The model under review builds one solid part; all positions refer to its coordinate system, in mm. Face numbers are marked on the shaded views. A direction names the side the tool comes from. Round coordinates to 2 decimals unless told otherwise and drop trailing zeros. Order: outer loops, then holes, each group sorted by start corner. A loop starts at its lowest first (then second) coordinate and runs counter-clockwise, first axis right, second up.
```python
from build123d import *

# Parameters (mm, degrees)
SKETCH1_R                   = 2.5
SKETCH1_R_2                 = 1
BOSS_EXTRUDE1_DEPTH         = 5
CHAMFER2_SIZE               = 4
CHAMFER2_SIZE2              = 0.705307923
LPATTERN2_COUNT             = 2
LPATTERN2_PITCH             = 5
CHAMFER2_OF_LPATTERN2_SIZE2 = 0.705307923
CHAMFER2_OF_LPATTERN2_SIZE  = 4
FILLET1_R                   = 1
SKETCH2_R                   = 10
BOSS_EXTRUDE2_DEPTH         = 15
CUT_EXTRUDE1_START          = -2
SKETCH3_R                   = 8
CUT_EXTRUDE1_DEPTH          = 15
CUT_EXTRUDE2_START          = -15
SKETCH4_R                   = 1
CUT_EXTRUDE2_DEPTH          = 15
FILLET2_R                   = 2
FILLET3_R                   = 2
FILLET4_R                   = 0.5
FILLET5_R                   = 0.5


with BuildPart() as part:
    # Sketch1 → Boss-Extrude1 (new body)
    with BuildSketch(Plane.XY):
        Circle(SKETCH1_R)
        Circle(SKETCH1_R_2, mode=Mode.SUBTRACT)
    boss_extrude1 = extrude(amount=BOSS_EXTRUDE1_DEPTH)

    # Chamfer2
    chamfer2_edges = [part.edges().sort_by_distance(p)[0] for p in [
        (-2.5, 0, 5),
    ]]
    chamfer2_side = [part.faces().sort_by_distance(p)[0] for p in [
        (-2.5, 0, 2.5),
    ]]
    chamfer(chamfer2_edges, length=CHAMFER2_SIZE, length2=CHAMFER2_SIZE2, reference=chamfer2_side[0])


with BuildPart() as lpattern2_1:
    # LPattern2: Boss-Extrude1 ×2
    with Locations(*[(0, 0, i * LPATTERN2_PITCH) for i in range(1, LPATTERN2_COUNT)]):
        add(boss_extrude1)

    # Chamfer2 of LPattern2
    chamfer2_of_lpattern2_edges = [lpattern2_1.edges().sort_by_distance(p)[0] for p in [
        (-2.5, 0, 10),
    ]]
    chamfer(chamfer2_of_lpattern2_edges, length=CHAMFER2_OF_LPATTERN2_SIZE, length2=CHAMFER2_OF_LPATTERN2_SIZE2)


with BuildPart() as part_1:
    add(part.part)

    # LPattern2 united with what the copies to: union LPattern2_1
    add(lpattern2_1.part)

    # Fillet1
    # the kernel refuses this fillet: 1 mm, written as the material it adds along each edge
    with BuildSketch(Plane(origin=(0, 0, 5), x_dir=(1, 0, 0), z_dir=(0, -1, 0))) as fillet1_piece_1:
        with BuildLine():
            CenterArc((2.96611905, -0.884722008), FILLET1_R, 117.782669079, 72.217330921)
            Line((1.981311297, -1.058370186), (1.961615141, -1.061843149))
            Line((1.961615141, -1.061843149), (1.774995922, -0.003472964))
            Line((1.774995922, -0.003472964), (1.794692077, 0.02))
            ThreePointArc((1.794692077, 0.02), (2.147346039, 0.02), (2.490677619, 0.01769444))
            Line((2.490677619, 0.01769444), (2.5, 0))
        make_face()
    revolve(axis=Axis((0, 0, 5), (0, 0, 1)))

    # Sketch2 → Boss-Extrude2 (add)
    with BuildSketch(Plane.XY):
        Circle(SKETCH2_R)
    extrude(amount=-BOSS_EXTRUDE2_DEPTH)

    # Sketch3 → Cut-Extrude1 (cut)
    with BuildSketch(Plane.XY.offset(CUT_EXTRUDE1_START)):
        Circle(SKETCH3_R)
    extrude(amount=-CUT_EXTRUDE1_DEPTH, mode=Mode.SUBTRACT)

    # Sketch4 → Cut-Extrude2 (cut)
    with BuildSketch(Plane.XY.offset(CUT_EXTRUDE2_START)):
        Circle(SKETCH4_R)
    extrude(amount=CUT_EXTRUDE2_DEPTH, mode=Mode.SUBTRACT)

    # Fillet2
    fillet2_edges = [part_1.edges().sort_by_distance(p)[0] for p in [
        (-1, 0, -2),
    ]]
    fillet(fillet2_edges, radius=FILLET2_R)

    # Fillet3
    fillet3_edges = [part_1.edges().sort_by_distance(p)[0] for p in [
        (-10, 0, 0),
    ]]
    fillet(fillet3_edges, radius=FILLET3_R)

    # Fillet4
    fillet4_edges = [part_1.edges().sort_by_distance(p)[0] for p in [
        (-2.5, 0, 0),
    ]]
    fillet(fillet4_edges, radius=FILLET4_R)

    # Fillet5
    fillet5_edges = [part_1.edges().sort_by_distance(p)[0] for p in [
        (-8, 0, -15),
    ]]
    fillet(fillet5_edges, radius=FILLET5_R)


solid = part_1.part
```
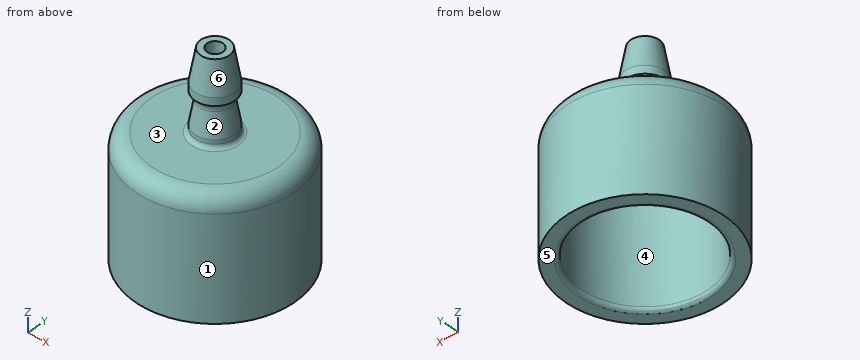
(1) Consider section C-C (z = -7). Write out the cut boundary in (x, y), and give its area (3 significant figures).
Data:
outline: circle Ø20 at (0, 0); hole circle Ø16 at (0, 0)
area: 113 mm2
(2) Consider section D-D (z = 4.5). Write out the cut boundary in (x, y).
Data:
outline: circle Ø4.09 at (0, 0); hole circle Ø2 at (0, 0)
(3) For the marked faces 1, 2 and 3, list the 3-axis set-ups (+Z, -Z, +X, -X, +Y, -Y) from which the entire face can be reached by the end or side of a thin tool; tool diameter is ignored.
Data:
face 1: +Z, -Z
face 2: none
face 3: +Z
(4) Insertion check: pin 1 (12 mm diameter, centred on x = -0.5, y = 3.5, fed in from -Z); pin 2 (1.2 mm diameter, centred on x = 0, y = 0, fed in from +Z); pin 3 (1.5 mm diameter, centred on x = -3.5, y = 4, fed in from -Z); pin 4 (4 mm diameter, centred on x = 3.5, z = -2.5, fed in from +Y). Each pin has a flat end and moves straight along its axis. Give the tip position at first contact, or say it passes through.
Data:
pin 1: stops at z = -15
pin 2: passes through
pin 3: stops at z = -2
pin 4: stops at y = 9.89
(5) To check wall thickness, follow probe 1 along Y at (x, z) = (0, -10); probe 2 along Z at (x, y) = (-3.5, 3); probe 3 along X at (y, z) = (-0.75, -6). State the ranges of each line that lie inside material, in increasing order.
Data:
probe 1: y = -10 to -8, 8 to 10
probe 2: z = -2 to 0
probe 3: x = -9.97 to -7.96, 7.96 to 9.97
(6) Draft analysis for pull direction Y (two halves, no side actions). For the marked faces 4, 5 and 6, state which applies: pulls with the +Y half, pulls with the -Y half, needs draft (parallel to the pull), parting line crosses it, or undercut.
Data:
face 4: undercut
face 5: needs draft
face 6: parting line crosses it
